Check sheet for the drawn part. Datum: minimum x, y, z corner. Units: mm. Coordinates: 2 decimals unless noted, no trailing zeros. Answer in a Markdown table with one row per item. Add a question column.
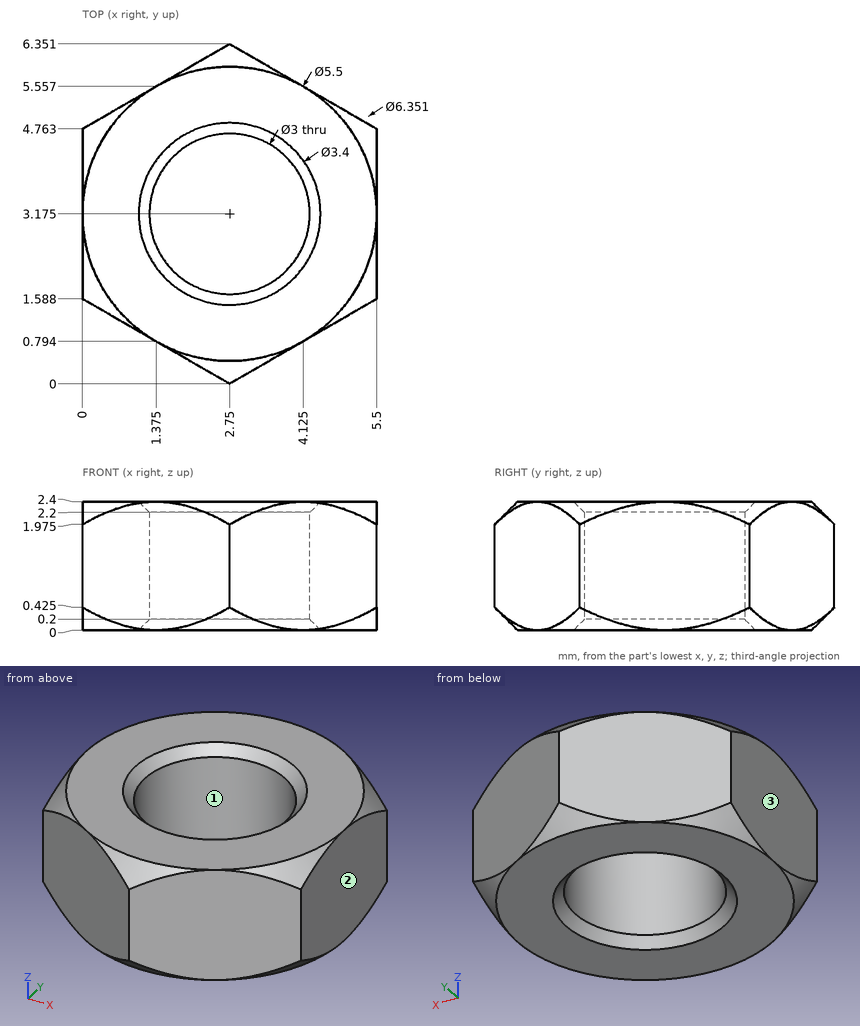
1. Release check for a two-part mould opening along X. For the marked faces 1, 2 and 3 record: released by +X, released by -X, zero draft, split by the parting line, or undercut.
2. Scan lines: line 1 (Y direction, x = 2, z = 2.25) (1 decimal); line 2 (Y direction, x = 1.65, z = 0.7) (1 decimal); line 3 (X direction, y = 2.5, z = 2.05). Record each from-to range of solid material in increasing order.
3. Go/stop test with a flat-tipped pin: pin 1 Ø2.5 at (x, y) = (2.75, 3.18) entering from -Z. Record where the tip stops, or that it passes through.
Result sheet:
| question | item | result |
|---|---|---|
| 1 | face 1 | undercut |
| 1 | face 2 | released by +X |
| 1 | face 3 | released by -X |
| 2 | line 1 | 0.4 to 1.8, 4.5 to 5.9 |
| 2 | line 2 | 0.6 to 2.2, 4.2 to 5.7 |
| 2 | line 3 | 0 to 1.41, 4.09 to 5.5 |
| 3 | pin 1 | through |
